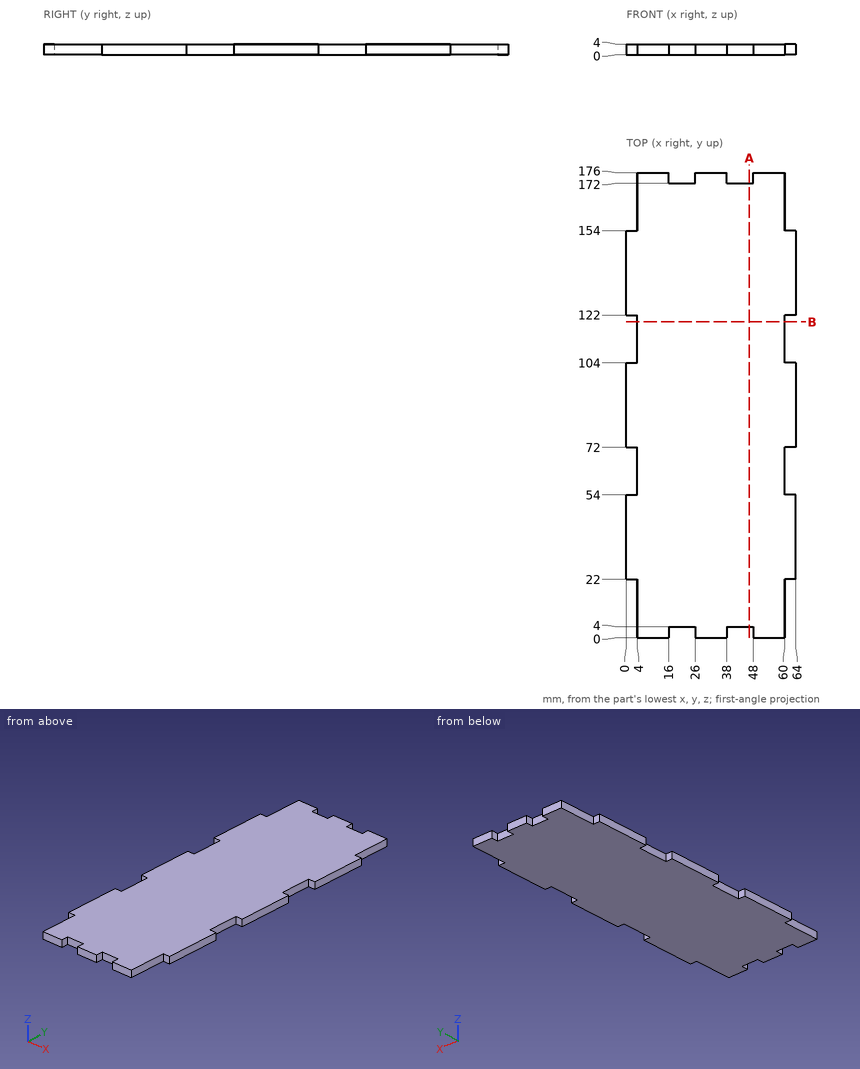
Check sheet for the drawn part. Datum: minimum x, y, z corner. Units: mm. Round coordinates to 2 decimals unless told otherwise and drop trailing zeros. Write each loop counter-clockwise with the first axis right and the second up, starting at its lowest first coordinate (ties: lowest second). Pieces come first, ordered by that corner, then holes. Notation, with made-up numbers: (34.5, -5) -> (91.5, -5) arc R13 cw to (91.5, 0) -> close; hole circle Ø3 at (54, -11.75). An arc over 180 degrees is marked (long way). One line per item, written item: value. Start each with the question number.
(1) Go/stop test with flat-tipped pins: pin 1 Ø2 at (y, z) = (60, 1) entering from -X; pin 2 Ø1.2 at (y, z) = (2.5, 1.5) entering from +X; pin 3 Ø1.2 at (x, z) = (20.5, 1) entering from -Y. Record where each tip stops, or that it passes through.
(2) Cross-section at A-A, the plane x = 46.5. Record the cut outline in (y, z), and give its area (3 significant figures).
(3) Scan lines: line 1 (X direction, y = 62, z = 2.9); line 2 (Y direction, x = 45, z = 1.65). Record each from-to range of solid material in increasing order. Write a range as [from, to].
(4) Cross-section at B-B, the plane y = 119.5. Record the cut outline in (x, z).
Answer:
1. pin 1: x = 4
1. pin 2: x = 60
1. pin 3: y = 4
2. outline: (4, 0) -> (172, 0) -> (172, 4) -> (4, 4) -> close
2. area: 672 mm²
3. line 1: [4, 60]
3. line 2: [4, 172]
4. outline: (4, 0) -> (60, 0) -> (60, 4) -> (4, 4) -> close
